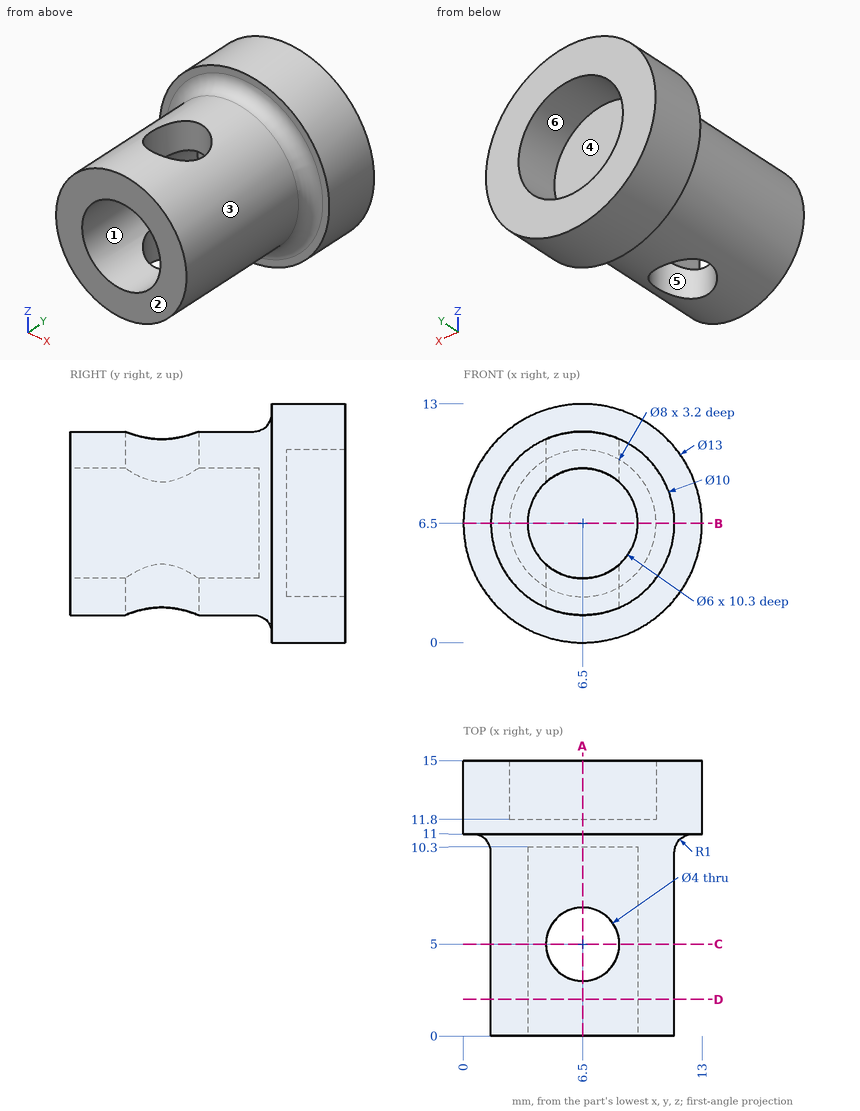
Could you check a few things on this drawing? It's one solid part, dimensions in mm from its lowest x, y, z. A direction names the side the tool comes from. Coordinates: 2 decimals unless noted, no trailing zeros. Order: outer loops, then holes, each group sorted by start corner. A loop starts at its lowest first (then second) coordinate and runs counter-clockwise, first axis right, second up. Notation, with made-up numbers: (20.5, 86.5) -> (36.5, 86.5) arc R13 ccw to (36.5, 90.5) -> close; hole circle Ø6 at (-19, 33.5). An arc over 180 degrees is marked (long way). Answer in a Markdown table with one row per item.
(1) I want a section at D-D on y = 2. List the corners of the cut face in (x, z) for me.
Answer key:
| item | result |
|---|---|
| outline | circle Ø10 at (6.5, 6.5); hole circle Ø6 at (6.5, 6.5) |
(2) Thinking about a two-plate mould opening in Z: for the marked faces 1, 2, 3 and 4, which applies, +Z half, -Z half, draft (parallel to the pull), parting line (faces both ways), or undercut?
Answer key:
| item | result |
|---|---|
| face 1 | undercut |
| face 2 | draft |
| face 3 | parting line |
| face 4 | undercut |
(3) Please list where these lines run through material, in increasing order: probe 1 along Z at (x, y) = (6.5, 13.8); probe 2 along Y at (x, z) = (6.5, 2.6); probe 3 along X at (y, z) = (6.75, 5.5).
Answer key:
| item | result |
|---|---|
| probe 1 | 0 to 2.5, 10.5 to 13 |
| probe 2 | 0 to 3, 7 to 11.8 |
| probe 3 | 1.6 to 3.67, 9.33 to 11.4 |
(4) On a 3-axis mill with a long thin cutter (end or side, diameter ignored), from which of +Z, -Z, +X, -X, +Y, -Y can I reach the whole of each face in a straight line? I mean the marked faces 5 and 6. Say none if no direction works.
Answer key:
| item | result |
|---|---|
| face 5 | +Z, -Z |
| face 6 | +Y |
(5) I want a section at B-B on z = 6.5. List the corners of the cut face in (x, y) for me.
Answer key:
| item | result |
|---|---|
| outline | (0, 11) -> (0.5, 11) arc R1 cw to (1.5, 10) -> (1.5, 0) -> (3.5, 0) -> (3.5, 10.3) -> (9.5, 10.3) -> (9.5, 0) -> (11.5, 0) -> (11.5, 10) arc R1 cw to (12.5, 11) -> (13, 11) -> (13, 15) -> (10.5, 15) -> (10.5, 11.8) -> (2.5, 11.8) -> (2.5, 15) -> (0, 15) -> close |
(6) I want a section at C-C on y = 5. List the corners of the cut face in (x, z) for me, then the cut area to 3 significant figures.
Answer key:
| item | result |
|---|---|
| outline | (4.5, 1.92) -> (4.5, 4.26) arc R3 cw to (4.5, 8.74) -> (4.5, 11.08) arc R5 ccw to start; (8.5, 1.92) arc R5 ccw to (8.5, 11.08) -> (8.5, 8.74) arc R3 cw to (8.5, 4.26) -> close |
| area | 33.4 mm^2 |
(7) Will these pins go through, and if not, where does the flat tip stop? pin 1 Ø1.5 at (x, y) = (7.5, 11.5) entering from -Z; pin 2 Ø6 at (x, y) = (11, 11) entering from +Z; pin 3 Ø4 at (y, z) = (5.5, 10) entering from -X.
Answer key:
| item | result |
|---|---|
| pin 1 | z = 0 |
| pin 2 | z = 12.82 |
| pin 3 | x = 1.73 |
(8) I want a section at A-A on x = 6.5. List the corners of the cut face in (y, z) for me.
Answer key:
| item | result |
|---|---|
| outline | (0, 1.5) -> (3, 1.5) -> (3, 3.5) -> (0, 3.5) -> close; (0, 9.5) -> (3, 9.5) -> (3, 11.5) -> (0, 11.5) -> close; (7, 1.5) -> (10, 1.5) arc R1 cw to (11, 0.5) -> (11, 0) -> (15, 0) -> (15, 2.5) -> (11.8, 2.5) -> (11.8, 10.5) -> (15, 10.5) -> (15, 13) -> (11, 13) -> (11, 12.5) arc R1 cw to (10, 11.5) -> (7, 11.5) -> (7, 9.5) -> (10.3, 9.5) -> (10.3, 3.5) -> (7, 3.5) -> close |
